Geometry check sheet. Reference: the model listing, model coordinates, mm. A direction names the side the tool comes from. Give positions to 0.01 mm unless a question says otherwise; leave off trailing zeros. Order: outer loops, then holes, each group sorted by start corner. A loop starts at its lowest first (then second) coordinate and runs counter-clockwise, first axis right, second up.
from build123d import *

# Parameters (mm, degrees)
SKETCH_1_W          = 100
SKETCH_1_H          = 30
EXTRUDE_1_DEPTH     = 20
EXTRUDE_2_DEPTH     = 25
FILLET_2_R          = 5
CUT_EXTRUDE_START   = -8
CUT_EXTRUDE_1_DEPTH = 8
SKETCH_5_R          = 1.5
CUT_EXTRUDE_2_DEPTH = 95.750127505


with BuildPart() as part:
    # 草图1 → 凸台-拉伸1 (new body)
    with BuildSketch(Plane.XY):
        with Locations((10, 0)):
            Rectangle(SKETCH_1_W, SKETCH_1_H)
    extrude(amount=EXTRUDE_1_DEPTH)

    # 草图2 → 凸台-拉伸2 (add)
    with BuildSketch(Plane.XY.offset(20)):
        with BuildLine():
            Line((60, 15), (70, 15))
            Line((70, 15), (90, -4))
            Line((90, -4), (90, -20))
            Line((90, -20), (90, -24.260805059))
            Line((90, -24.260805059), (77.430397402, -20.975197102))
            ThreePointArc((77.430397402, -20.975197102), (73.668164046, -20.244798043), (69.843512882, -20))
            Line((69.843512882, -20), (60, -20))
            Line((60, -20), (60, 15))
        make_face()
    extrude(amount=-EXTRUDE_2_DEPTH)

    # 圆角2
    fillet_2_edges = [part.edges().sort_by_distance(p)[0] for p in [
        (60, -15, 10),
        (60, 0, 0),
    ]]
    fillet(fillet_2_edges, radius=FILLET_2_R - 0.0001)  # a hair under: the kernel refuses the full size

    # 草图4 → 切除-拉伸1 (cut)
    with BuildSketch(Plane(origin=(0, 0, -5), x_dir=(-1, 0, 0), z_dir=(0, 0, -1)).offset(CUT_EXTRUDE_START)):
        with BuildLine():
            Line((-90, -8.096027328), (-75, -8.928770232))
            Line((-75, -8.928770232), (-75, -20.446478372))
            ThreePointArc((-75, -20.446478372), (-76.220680439, -20.685639459), (-77.430397402, -20.975197102))
            Line((-77.430397402, -20.975197102), (-90, -24.260805059))
            Line((-90, -24.260805059), (-90, -8.096027328))
        make_face()
    extrude(amount=CUT_EXTRUDE_1_DEPTH, mode=Mode.SUBTRACT)

    # 草图5 → 切除-拉伸2 (cut, through all)
    with BuildSketch(Plane(origin=(0, 0, 3), x_dir=(-1, 0, 0), z_dir=(0, 0, -1))):
        with Locations((-81.993244167, -16.076814441)):
            Circle(SKETCH_5_R)
    extrude(amount=-CUT_EXTRUDE_2_DEPTH, mode=Mode.SUBTRACT)


solid = part.part
Item 1: Gauge pin test, flat ends, axial feed: pin 1 (2 mm diameter, centred on x = 58.5, z = -2.5, fed in from -Y); pin 2 (4.5 mm diameter, centred on x = 81.5, y = -16, fed in from -Z); pin 3 (4 mm diameter, centred on y = -12, z = -0.5, fed in from +X); pin 4 (2.5 mm diameter, centred on x = 81.99, y = -16.08, fed in from +Z). Record the tip position at first contact, or that the pin passes through.
Reported:
pin 1: stops at y = -17.82
pin 2: stops at z = 3
pin 3: stops at x = 75
pin 4: passes through
Item 2: Sectioned sample at C-C (x = -16). Enter the section's corners in (y, z).
Reported:
outline: (-15, 0) - (15, 0) - (15, 20) - (-15, 20) - close
Item 3: Draft check along X on faces 1 (the cylindrical face through (83.184, -16.99, 11.381)), 2 (the flat face through (75, -15, -1)), 3 (the cylindrical face through (58, -16, 10)), 4 (the flat face through (26, 0, 20)). Enter one of: released by +X, released by -X, zero draft, split by the parting line, or undercut.
Reported:
face 1: undercut
face 2: released by +X
face 3: released by -X
face 4: zero draft
Item 4: Set-up check for faces 5 (the flat face through (7, 0, 0)), 6 (the flat face through (7, -15, 10)), 7 (the flat face through (79.86, 5.633, 7.675)), 8 (the flat face through (82, -14, 3)), 9 (the flat face through (-40, 0, 10)): record each of +Z, -Z, +X, -X, +Y, -Y from which the full face is reachable in a straight line by a thin tool's end or side.
Reported:
face 5: -Z, -X, +Y, -Y
face 6: +Z, -Z, -X, -Y
face 7: +Z, -Z, +X, +Y
face 8: -Z, +X, -Y
face 9: +Z, -Z, -X, +Y, -Y
Item 5: Scan lines: L1, parallel to Y at x = 3.5, z = 10; L2, parallel to Z at x = 15, y = -13; L3, parallel to X at y = 12.5, z = 3.5. Record each from-to range of solid material in increasing order.
Reported:
L1: y = -15 to 15
L2: z = 0 to 20
L3: x = -40 to 72.63
